Check sheet for the drawn part. Datum: minimum x, y, z corner. Units: mm. A direction names the side the tool comes from. Coordinates: 2 decimals unless noted, no trailing zeros. Order: outer loops, then holes, each group sorted by start corner. A loop starts at its lowest first (then second) coordinate and runs counter-clockwise, first axis right, second up.
1. Draft check along X on the marked faces 3, 4 and 5. Enter one of: released by +X, released by -X, zero draft, split by the parting line, or undercut.
2. Thickness scan on line 1 (Y direction, x = 6, z = 28); line 2 (X direction, y = 3.5, z = 24); line 3 (Z direction, x = 6, y = 7.25). Record the ranges inside material, lowest first.
3. Gauge pin test, flat ends, axial feed: pin 1 Ø6 at (x, y) = (6, 9.5) entering from -Z; pin 2 Ø7 at (y, z) = (10.5, 30) entering from +X; pin 3 Ø8 at (y, z) = (11, 5) entering from +X. Record the tip position at first contact, or that the pin passes through.
4. Cross-section at D-D (y = 1). Enter the section's corners in (x, z), then the cut area to 3 significant figures.
5. Cross-section at C-C (x = 2). Enter the section's corners in (y, z), then the cut area to 3 significant figures.
6. Cross-section at A-A (y = 7.5). Enter the section's corners in (x, z).
7. Cross-section at B-B (z = 28). Enter the section's corners in (x, y), then the cut area to 3 significant figures.
8. Set-up check for the marked faces 1 and 2: record each of +Z, -Z, +X, -X, +Y, -Y from which the full face is reachable in a straight line by a thin tool's end or side.
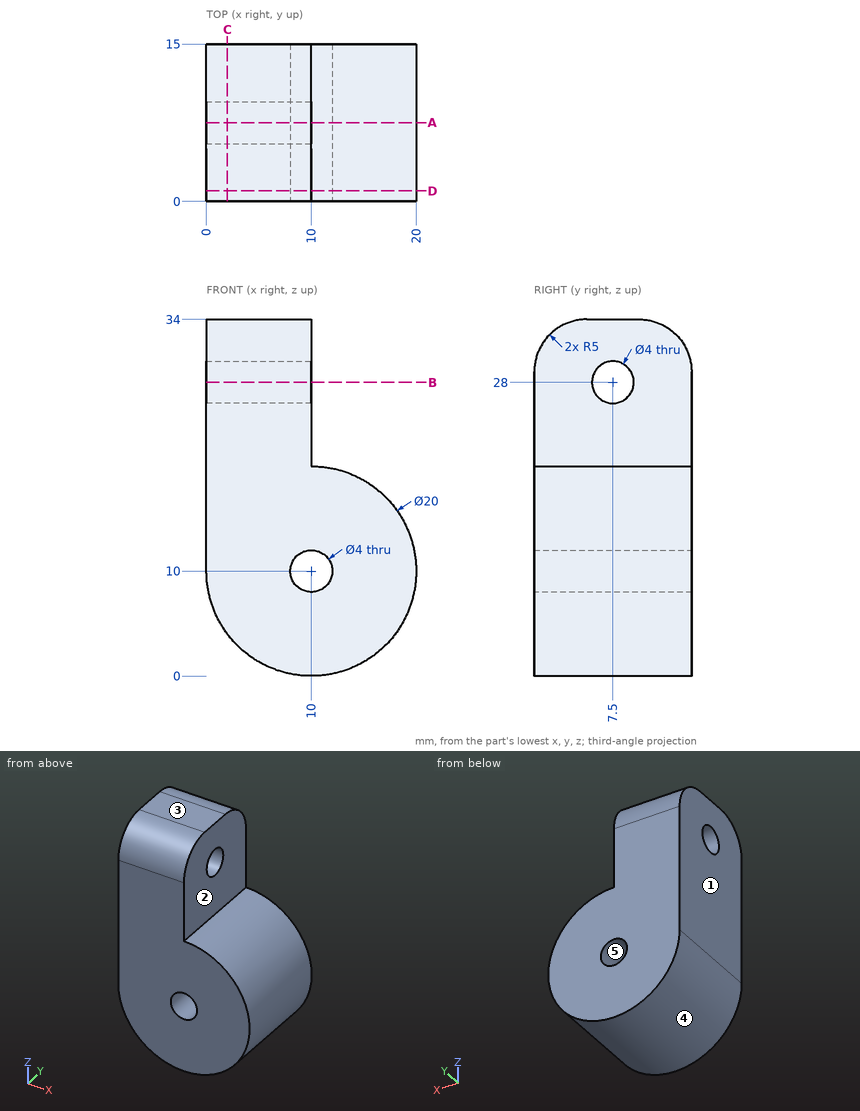
Data:
1. face 3: zero draft
1. face 4: split by the parting line
1. face 5: undercut
2. line 1: y = 0 to 5.5, 9.5 to 15
2. line 2: x = 0 to 10
2. line 3: z = 0.83 to 26.02, 29.98 to 34
3. pin 1: stops at z = 0.05
3. pin 2: stops at x = 10
3. pin 3: stops at x = 19.95
4. outline: (0, 10) arc R10 ccw (long way) to (10, 20) - (10, 32) - (0, 32) - close; hole circle Ø4 at (10, 10)
4. area: 443 mm2
5. outline: (0, 4) - (15, 4) - (15, 29) arc R5 ccw to (10, 34) - (5, 34) arc R5 ccw to (0, 29) - close; hole circle Ø4 at (7.5, 28)
5. area: 427 mm2
6. outline: (0, 10) arc R10 ccw (long way) to (10, 20) - (10, 26) - (0, 26) - close; (0, 30) - (10, 30) - (10, 34) - (0, 34) - close; hole circle Ø4 at (10, 10)
7. outline: (0, 0) - (10, 0) - (10, 5.5) - (0, 5.5) - close; (0, 9.5) - (10, 9.5) - (10, 15) - (0, 15) - close
7. area: 110 mm2
8. face 1: +Z, -Z, -X, +Y, -Y
8. face 2: +Z, +X, +Y, -Y
